The model under review builds one solid part; all positions refer to its coordinate system, in mm. Face numbers are marked on the shaded views. Round coordinates to 2 decimals unless told otherwise and drop trailing zeros. Write each loop counter-clockwise with the first axis right and the second up, starting at its lowest first coordinate (ties: lowest second). Pieces come first, ordered by that corner, then holes. Notation, with made-up numbers: (23.25, 14) - (47.25, 14) arc R12 cw to (47.25, 32) - close; hole circle Ø3 at (3.25, -40). An arc over 180 degrees is marked (long way). Use one line per item in the form item = value.
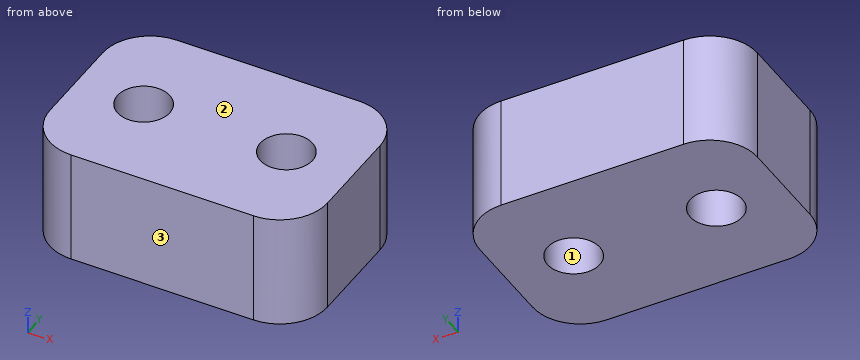
from build123d import *

# Parameters (mm, degrees)
SKETCH1_W           = 17.5
SKETCH1_H           = 12
BOSS_EXTRUDE1_DEPTH = 7.2
FILLET1_R           = 3
SKETCH2_R           = 1.65
CUT_EXTRUDE1_DEPTH  = 8.2


with BuildPart() as part:
    # Sketch1 → Boss-Extrude1 (new body)
    with BuildSketch(Plane.XY):
        Rectangle(SKETCH1_W, SKETCH1_H)
    extrude(amount=BOSS_EXTRUDE1_DEPTH)

    # Fillet1
    fillet1_edges = [part.edges().sort_by_distance(p)[0] for p in [
        (-8.75, 6, 3.6),
        (8.75, 6, 3.6),
        (8.75, -6, 3.6),
        (-8.75, -6, 3.6),
    ]]
    fillet(fillet1_edges, radius=FILLET1_R)

    # Sketch2 → Cut-Extrude1 (cut, through all)
    with BuildSketch(Plane.XY.offset(7.2)):
        with Locations((-4.5, 0)):
            Circle(SKETCH2_R)
        with Locations((4.5, 0)):
            Circle(SKETCH2_R)
    extrude(amount=-CUT_EXTRUDE1_DEPTH, mode=Mode.SUBTRACT)


solid = part.part
(1) Insertion check: P1, Ø1.5, axis at y = -4, z = 1, coming from the -X side. The pin has a flat end and moves straight along its axis. Give the tip position at first contact, or say it passes through.
Geometry results:
P1 = -8.74
(2) The part is to be moulded in two halves that separate along Y. For the marked faces 1, 2 and 3, say which applies: +Y half, -Y half, draft (parallel to the pull), parting line (faces both ways), or undercut.
Geometry results:
face_1 = undercut
face_2 = draft
face_3 = -Y half
(3) Add section B-B on y = 0. Write out the cut boundary in (x, z).
Geometry results:
outline = (-8.75, 0) - (-6.15, 0) - (-6.15, 7.2) - (-8.75, 7.2) - close; (-2.85, 0) - (2.85, 0) - (2.85, 7.2) - (-2.85, 7.2) - close; (6.15, 0) - (8.75, 0) - (8.75, 7.2) - (6.15, 7.2) - close
(4) Add section C-C on z = 4.25. Write out the cut boundary in (x, y), then the cut area to 3 significant figures.
Geometry results:
outline = (-8.75, -3) arc R3 ccw to (-5.75, -6) - (5.75, -6) arc R3 ccw to (8.75, -3) - (8.75, 3) arc R3 ccw to (5.75, 6) - (-5.75, 6) arc R3 ccw to (-8.75, 3) - close; hole circle Ø3.3 at (-4.5, 0); hole circle Ø3.3 at (4.5, 0)
area = 185 mm2
(5) Add section A-A on x = 4.5. Write out the cut boundary in (y, z), then the cut area to 3 significant figures.
Geometry results:
outline = (-6, 0) - (-1.65, 0) - (-1.65, 7.2) - (-6, 7.2) - close; (1.65, 0) - (6, 0) - (6, 7.2) - (1.65, 7.2) - close
area = 62.6 mm2
(6) To check wall thickness, follow L1, parallel to Y at x = -4.5, z = 3; L2, parallel to X at y = 1, z = 5.5; L3, parallel to Y at x = 6, z = 1.5. State the ranges of each line that lie inside material, in increasing order.
Geometry results:
L1 = -6 to -1.65, 1.65 to 6
L2 = -8.75 to -5.81, -3.19 to 3.19, 5.81 to 8.75
L3 = -5.99 to -0.69, 0.69 to 5.99
(7) Add section D-D on x = -4.75. Write out the cut boundary in (y, z), then the cut area to 3 significant figures.
Geometry results:
outline = (-6, 0) - (-1.63, 0) - (-1.63, 7.2) - (-6, 7.2) - close; (1.63, 0) - (6, 0) - (6, 7.2) - (1.63, 7.2) - close
area = 62.9 mm2
